from build123d import *

# Parameters (mm, degrees)
BOSS_EXTRUDE1_DEPTH     = 63.5
F_1_4_CLEARANCE_HOLE1_D = 7.14248
F_1_4_CLEARANCE_HOLE2_D = 7.14248
CHAMFER4_SIZE           = 6.35


with BuildPart() as part:
    # Sketch1 → Boss-Extrude1 (new body)
    with BuildSketch(Plane.XY):
        Polygon((0, 0), (38.1, 0), (38.1, 25.4), (33.3375, 25.4), (33.3375, 4.7625), (0, 4.7625), align=None)
    boss_extrude1 = extrude(amount=BOSS_EXTRUDE1_DEPTH)

    # 1/4 Clearance Hole1 (through all)
    with Locations(Plane(origin=(0, 4.7625, 0), x_dir=(1, 0, 0), z_dir=(0, 1, 0))):
        with Locations((12.7, -12.7), (12.7, -38.1)):
            f_1_4_clearance_hole1 = Hole(F_1_4_CLEARANCE_HOLE1_D / 2)

    # 1/4 Clearance Hole2 (through all)
    with Locations(Plane.ZY.offset(-33.3375)):
        with Locations((38.1, 12.7), (12.7, 12.7)):
            f_1_4_clearance_hole2 = Hole(F_1_4_CLEARANCE_HOLE2_D / 2)

    # Mirror1: Boss-Extrude1, 1/4 Clearance Hole1, 1/4 Clearance Hole2 across plane
    add(boss_extrude1.mirror(Plane(origin=(-12.7, 0, 12.7), x_dir=(0.7071067811865477, 0, 0.7071067811865474), z_dir=(0.7071067811865474, 0, -0.7071067811865477))))
    add(f_1_4_clearance_hole1.mirror(Plane(origin=(-12.7, 0, 12.7), x_dir=(0.7071067811865477, 0, 0.7071067811865474), z_dir=(0.7071067811865474, 0, -0.7071067811865477))), mode=Mode.SUBTRACT)
    add(f_1_4_clearance_hole2.mirror(Plane(origin=(-12.7, 0, 12.7), x_dir=(0.7071067811865477, 0, 0.7071067811865474), z_dir=(0.7071067811865474, 0, -0.7071067811865477))), mode=Mode.SUBTRACT)

    # Chamfer4
    chamfer4_edges = [part.edges().sort_by_distance(p)[0] for p in [
        (-25.4, 2.38125, 25.4),
        (0, 2.38125, 0),
    ]]
    chamfer(chamfer4_edges, length=CHAMFER4_SIZE)


solid = part.part
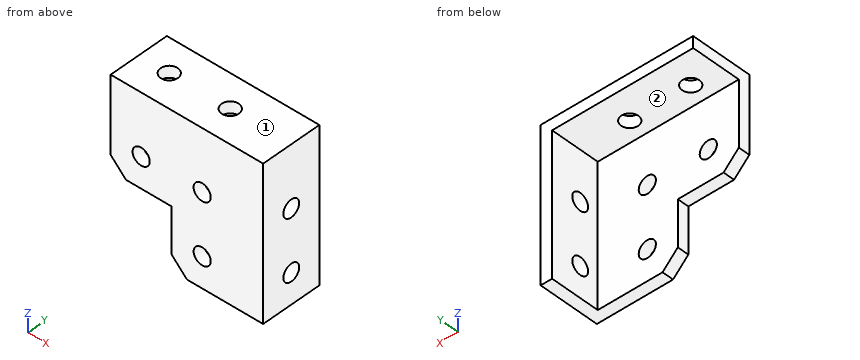
Build history of the part. All positions in model axes, mm. Face numbers are marked on the shaded views. A direction names the side the tool comes from. Give positions to 0.01 mm unless a question says otherwise; leave off trailing zeros. Order: outer loops, then holes, each group sorted by start corner. A loop starts at its lowest first (then second) coordinate and runs counter-clockwise, first axis right, second up. Notation, with made-up numbers: M 16.5,61.25 L 66.5,61.25 A8 ccw 66.5,69.25 Z; hole C 88.25,-10.5 d11. An arc over 180 degrees is marked long. Use one line per item in the form item = value.
1) Saw through at C-C (z = 12.7). Give the cut face in (x, y).
Calculated:
outline = M 0,0 L 9.13,0 L 9.13,4.76 L 0,4.76 Z; M 16.27,0 L 38.1,0 L 38.1,9.13 L 33.34,9.13 L 33.34,4.76 L 16.27,4.76 Z; M 33.34,16.27 L 38.1,16.27 L 38.1,25.4 L 33.34,25.4 Z
2) Saw through at A-A (x = -12.7). Give the cut face in (y, z).
Calculated:
outline = M 0,25.4 L 4.76,25.4 L 4.76,34.53 L 0,34.53 Z; M 0,41.67 L 4.76,41.67 L 4.76,58.74 L 9.13,58.74 L 9.13,63.5 L 0,63.5 Z; M 16.27,58.74 L 25.4,58.74 L 25.4,63.5 L 16.27,63.5 Z
3) Saw through at D-D (z = 38.1). Give the cut face in (x, y), plus the area to 3 significant figures.
Calculated:
outline = M -25.4,0 L -16.27,0 L -16.27,4.76 L -25.4,4.76 Z; M -9.13,0 L 9.13,0 L 9.13,4.76 L -9.13,4.76 Z; M 16.27,0 L 38.1,0 L 38.1,9.13 L 33.34,9.13 L 33.34,4.76 L 16.27,4.76 Z; M 33.34,16.27 L 38.1,16.27 L 38.1,25.4 L 33.34,25.4 Z
area = 299 mm2
4) Saw through at B-B (y = 12.7). Give the cut face in (x, z).
Calculated:
outline = M -25.4,58.74 L -16.27,58.74 L -16.27,63.5 L -25.4,63.5 Z; M -9.13,58.74 L 9.13,58.74 L 9.13,63.5 L -9.13,63.5 Z; M 16.27,58.74 L 33.34,58.74 L 33.34,41.67 L 38.1,41.67 L 38.1,63.5 L 16.27,63.5 Z; M 33.34,0 L 38.1,0 L 38.1,9.13 L 33.34,9.13 Z; M 33.34,16.27 L 38.1,16.27 L 38.1,34.53 L 33.34,34.53 Z
5) Probe probe 1 along X at (y, z) = (12.7, 60.95); probe 2 along Y at (x, z) = (35.5, 12.7); probe 3 along X at (y, z) = (13.25, 59). List the from-to ranges inside material, lowest first.
Calculated:
probe_1 = -25.4 to -16.27, -9.13 to 9.13, 16.27 to 38.1
probe_2 = 0 to 9.13, 16.27 to 25.4
probe_3 = -25.4 to -16.23, -9.17 to 9.17, 16.23 to 38.1
6) Drop flat-ended pins along their axis: pin 1 (12 mm diameter, centred on x = -18, z = 23.5, fed in from +Y); pin 2 (11.5 mm diameter, centred on y = 12.7, z = 38.1, fed in from -X); pin 3 (8 mm diameter, centred on x = 12.7, z = 38.1, fed in from -Y); pin 4 (3 mm diameter, centred on x = 19.5, y = 20, fed in from -Z). Give the stop position or say it passes through.
Calculated:
pin_1 = 4.76
pin_2 = 33.34
pin_3 = 0
pin_4 = 58.74
7) Tool access for the marked faces 1 and 2: list every direction of +Z, -Z, +X, -X, +Y, -Y with a clear straight run to the whole face (end or side of a thin tool).
Calculated:
face_1 = +Z, +X, -X, +Y, -Y
face_2 = -Z, -X, +Y
